Read the model definition and answer for the solid it produces. Units are mm, in the model's axes. A direction names the side the tool comes from. Give positions to 0.01 mm unless a question says otherwise; leave off trailing zeros. Order: outer loops, then holes, each group sorted by start corner. A loop starts at its lowest first (then second) coordinate and runs counter-clockwise, first axis right, second up. Notation, with made-up numbers: (81, 58) -> (135, 58) arc R30 cw to (135, 95) -> close; hole circle Ø5 at (-15, 67). An arc over 180 degrees is marked (long way). Use one line per item in the form item = value.
```python
from build123d import *

# Parameters (mm, degrees)
F0_W     = 114
F0_H     = 190
F1_DEPTH = 25
F2_R     = 5
F3_T     = -3


with BuildPart() as f1:
    # F0 (on Front) → F1 (new body)
    with BuildSketch(Plane.XZ):
        Rectangle(F0_W, F0_H)
    extrude(amount=F1_DEPTH)

    # F2
    f2_edges = [f1.edges().sort_by_distance(p)[0] for p in [
        (57, -12.5, -95),
        (-57, -12.5, -95),
    ]]
    fillet(f2_edges, radius=F2_R)

    # F3
    f3_openings = [f1.faces().sort_by_distance(p)[0] for p in [
        (0, -25, 0.046532),
        (0, -12.5, 95),
    ]]
    offset(amount=F3_T, openings=f3_openings)


solid = f1.part
```
Item 1: Given pin 1 Ø3 at (x, z) = (2, 42.5) entering from -Y; pin 2 Ø6 at (x, y) = (2.5, -22) entering from +Z, each flat-ended and moving along its own axis, determine where each tip first touches the part or whether it passes through.
Checks:
pin_1 = -3
pin_2 = -92
Item 2: Determine the mould class of faces 1 (the flat face through (0, -2, 95)), 2 (the cylindrical face through (55, -13, -94)), 3 (the flat face through (54, -14, 1)), 4 (the flat face through (-1, -3, 3)) for opening direction X: +X half, -X half, draft (parallel to the pull), parting line (faces both ways), or undercut.
Checks:
face_1 = draft
face_2 = +X half
face_3 = undercut
face_4 = undercut
Item 3: The part is cut by section B-B on x = 46.5. Give the vertices of the cut face in (y, z), and give its area (3 significant figures).
Checks:
outline = (-25, -95) -> (0, -95) -> (0, 95) -> (-3, 95) -> (-3, -92) -> (-25, -92) -> close
area = 636 mm²
Item 4: Which of the six approach directions +Z, -Z, +X, -X, +Y, -Y give full straight-line access (tool end or side, diameter ignored) to faces 5 (the flat face through (-1, -12, -95)), 6 (the flat face through (-54, -14, 1))?
Checks:
face_5 = -Z, +X, -X, +Y, -Y
face_6 = +Z, -Y
Item 5: The part is cut by section C-C on z = 9. Give the vertices of the cut face in (x, y).
Checks:
outline = (-57, -25) -> (-54, -25) -> (-54, -3) -> (54, -3) -> (54, -25) -> (57, -25) -> (57, 0) -> (-57, 0) -> close
Item 6: Straight lines are drawn through the part: L1, parallel to X at y = -21.5, z = 9; L2, parallel to Z at x = -4.5, y = -14.25; L3, parallel to Y at x = -3.5, z = -4.5. For each, find the intervals that lie inside material, in ascending order. Write a range as from..to.
Checks:
L1 = -57..-54, 54..57
L2 = -95..-92
L3 = -3..0
Item 7: The part is cut by section A-A on y = -21.5. Give the vertices of the cut face in (x, z).
Checks:
outline = (-57, -90) arc R5 ccw to (-52, -95) -> (52, -95) arc R5 ccw to (57, -90) -> (57, 95) -> (54, 95) -> (54, -90) arc R2 cw to (52, -92) -> (-52, -92) arc R2 cw to (-54, -90) -> (-54, 95) -> (-57, 95) -> close
